Read the model definition and answer for the solid it produces. Units are mm, in the model's axes. A direction names the side the tool comes from. Give positions to 0.01 mm unless a question says otherwise; leave off trailing zeros. Loops run counter-clockwise (first coordinate to the right, second up) from the corner with the lowest first, then second, coordinate; pieces in that order, holes last.
(1) Determine the mould class of faces 4 (the face through (12, 1, -1.5)), 5 (the face through (11.5, 1, 0)), 6 (the face through (-0.33, 4.479, 7.493)) for opening direction X: pulls with the +X half, pulls with the -X half, needs draft (parallel to the pull), parting line crosses it, or undercut.
(2) Find section D-D, the plane y = 2.25. Write down the section's boundary in (x, z), then the cut area to 3 significant figures.
(3) Each of these flat-tipped pins is pushed along its axis until it touches: P1, Ø0.9, axis at y = 0.5, z = 0, coming from the +X side; P2, Ø1.5, axis at y = 3, z = 0.5, coming from the -X side; P3, Ø6, axis at x = 3.5, z = -7, coming from the -Y side; P4, Ø6, axis at x = -9.5, z = 2.5, coming from the -Y side. Where does it stop, or does it pass through?
(4) Find section B-B, the plane y = -0.5. Write down the section's boundary in (x, z).
(5) Find section C-C, the plane x = 0. Write down the section's boundary in (y, z), then the cut area to 3 significant figures.
(6) Straight lines are drawn through the part: probe 1 along X at (y, z) = (3.5, 0); probe 2 along Z at (x, y) = (0, 0.6); probe 3 along X at (y, z) = (2, 0.25). For each, find the intervals that lie inside material, in ascending order.
(7) Find section A-A, the plane z = 0. Write down the section's boundary in (x, y).
(8) Which of the six approach directions +Z, -Z, +X, -X, +Y, -Y give full straight-line access (tool end or side, diameter ignored) to faces 1 (the face through (12, 1, 1.5)), 2 (the face through (-12, 1, -1.5)), 3 (the face through (-2.914, 1.521, -9.252))?
```python
from build123d import *

# Parameters (mm, degrees)
SKETCH4_R          = 11.2
SKETCH4_R_2        = 9.7
CUT_EXTRUDE1_DEPTH = 2
CUT_EXTRUDE5_DEPTH = 20.661637775


with BuildPart() as part:
    # Sketch1 → Revolve1 (revolve)
    with BuildSketch(Plane.XY, mode=Mode.PRIVATE) as revolve1_sk:
        Polygon((-9.7, 0), (-9.7, -2), (-12.7, -2), (-12.7, 3.143703987), (-10.7, 6), (-7.5, 6), (-7.5, 3), (-9.7, 3), align=None)
    revolve(revolve1_sk.sketch.rotate(Axis((0, 0, 0), (0, 1, 0)), 270), axis=Axis((0, 0, 0), (0, 1, 0)))

    # Sketch4 → Cut-Extrude1 (cut)
    with BuildSketch(Plane.XZ.offset(2)):
        with Locations(Location((0, 0, 0), (0, 0, 270))):
            Circle(SKETCH4_R)
        with Locations(Location((0, 0, 0), (0, 0, 270))):
            Circle(SKETCH4_R_2, mode=Mode.SUBTRACT)
    extrude(amount=-CUT_EXTRUDE1_DEPTH, mode=Mode.SUBTRACT)

    # Sketch8 → Cut-Extrude5 (cut, through all)
    with BuildSketch(Plane(origin=(0, 6, 0), x_dir=(1, 0, 0), z_dir=(0, 1, 0))):
        with BuildLine():
            Line((-11.5, -1.5), (-11.5, 1.5))
            Line((-11.5, 1.5), (-12.611106216, 1.5))
            ThreePointArc((-12.611106216, 1.5), (-12.7, 0), (-12.611106216, -1.5))
            Line((-12.611106216, -1.5), (-11.5, -1.5))
        make_face()
        with BuildLine():
            Line((12.611106216, 1.5), (11.5, 1.5))
            Line((11.5, 1.5), (11.5, -1.5))
            Line((11.5, -1.5), (12.611106216, -1.5))
            ThreePointArc((12.611106216, -1.5), (12.677757076, -0.751315863), (12.7, 0))
            ThreePointArc((12.7, 0), (12.677757076, 0.751315863), (12.611106216, 1.5))
        make_face()
    extrude(amount=-CUT_EXTRUDE5_DEPTH, mode=Mode.SUBTRACT)


solid = part.part
```
Entries:
1. face 4: needs draft
1. face 5: pulls with the +X half
1. face 6: undercut
2. outline: (-12.61, -1.5) arc R12.7 ccw to (12.61, -1.5) - (11.5, -1.5) - (11.5, 1.5) - (12.61, 1.5) arc R12.7 ccw to (-12.61, 1.5) - (-11.5, 1.5) - (-11.5, -1.5) - close; hole circle Ø19.4 at (0, 0)
2. area: 204 mm2
3. P1: stops at x = 11.5
3. P2: stops at x = -11.5
3. P3: stops at y = 0
3. P4: stops at y = -2
4. outline: (-12.61, -1.5) arc R12.7 ccw to (12.61, -1.5) - (11.5, -1.5) - (11.5, 1.5) - (12.61, 1.5) arc R12.7 ccw to (-12.61, 1.5) - (-11.5, 1.5) - (-11.5, -1.5) - close; hole circle Ø22.4 at (0, 0)
5. outline: (-2, -12.7) - (3.14, -12.7) - (6, -10.7) - (6, -7.5) - (3, -7.5) - (3, -9.7) - (0, -9.7) - (0, -11.2) - (-2, -11.2) - close; (-2, 11.2) - (0, 11.2) - (0, 9.7) - (3, 9.7) - (3, 7.5) - (6, 7.5) - (6, 10.7) - (3.14, 12.7) - (-2, 12.7) - close
5. area: 49.5 mm2
6. probe 1: x = -11.5 to -7.5, 7.5 to 11.5
6. probe 2: z = -12.7 to -9.7, 9.7 to 12.7
6. probe 3: x = -11.5 to -9.7, 9.7 to 11.5
7. outline: (-11.5, -2) - (-11.2, -2) - (-11.2, 0) - (-9.7, 0) - (-9.7, 3) - (-7.5, 3) - (-7.5, 6) - (-10.7, 6) - (-11.5, 4.86) - close; (7.5, 3) - (9.7, 3) - (9.7, 0) - (11.2, 0) - (11.2, -2) - (11.5, -2) - (11.5, 4.86) - (10.7, 6) - (7.5, 6) - close
8. face 1: +X, +Y, -Y
8. face 2: -X, +Y, -Y
8. face 3: -Y
